```python
from build123d import *

# Parameters (mm, degrees)
F0_R     = 1.6002
F1_DEPTH = 6.35


with BuildPart() as f1:
    # F0 (on Right) → F1 (new body)
    with BuildSketch(Plane.YZ):
        Polygon((6.35, 0), (-6.35, 0), (-6.35, 6.604), (-21.59, 6.604), (-21.59, -19.304), (-6.35, -19.304), (-6.35, -12.7), (6.35, -12.7), (6.35, -19.304), (21.59, -19.304), (21.59, 6.604), (6.35, 6.604), align=None)
        with Locations((-6.35, -6.35)):
            Circle(F0_R, mode=Mode.SUBTRACT)
    extrude(amount=F1_DEPTH)


solid = f1.part
```
The model under review builds one solid part; all positions refer to its coordinate system, in mm. A direction names the side the tool comes from. Round coordinates to 2 decimals unless told otherwise and drop trailing zeros. Write each loop counter-clockwise with the first axis right and the second up, starting at its lowest first coordinate (ties: lowest second). Pieces come first, ordered by that corner, then holes. Notation, with made-up numbers: (30.5, 67.25) -> (57.5, 67.25) arc R10 cw to (57.5, 81.25) -> close; hole circle Ø1 at (68, -30). An arc over 180 degrees is marked (long way). Use CSV: the item, a comma, the result in double quotes.
Q1. Mouldability with a two-part tool opening along Y and no side actions: class faces 4 (the flat face through (3, 14, -19.304)), 5 (the flat face through (3, -6.35, 3)), 6 (the flat face through (3, 21.59, -7)) as released by +Y, released by -Y, zero draft, split by the parting line, or undercut.
Checks:
face 4,"zero draft"
face 5,"undercut"
face 6,"released by +Y"
Q2. Consider section C-C (y = 5). Give the boundary of the cut face in (x, z), then the cut area to 3 significant figures.
Checks:
outline,"(0, -12.7) -> (6.35, -12.7) -> (6.35, 0) -> (0, 0) -> close"
area,"80.6 mm²"
Q3. Consider section B-B (x = 5.75). Give the boundary of the cut face in (y, z).
Checks:
outline,"(-21.59, -19.3) -> (-6.35, -19.3) -> (-6.35, -12.7) -> (6.35, -12.7) -> (6.35, -19.3) -> (21.59, -19.3) -> (21.59, 6.6) -> (6.35, 6.6) -> (6.35, 0) -> (-6.35, 0) -> (-6.35, 6.6) -> (-21.59, 6.6) -> close; hole circle Ø3.2 at (-6.35, -6.35)"
Q4. Consider section A-A (z = 0.75). Give the boundary of the cut face in (x, y), then the cut area to 3 significant figures.
Checks:
outline,"(0, -21.59) -> (6.35, -21.59) -> (6.35, -6.35) -> (0, -6.35) -> close; (0, 6.35) -> (6.35, 6.35) -> (6.35, 21.59) -> (0, 21.59) -> close"
area,"194 mm²"
Q5. For pin 1 Ø3 at (x, y) = (4, 0.5) entering from +Z; pin 2 Ø1.9 at (x, y) = (2.5, 1.5) entering from -Z, all flat-tipped, find the tip position at first contact; note any pin that passes through.
Checks:
pin 1,"z = 0"
pin 2,"z = -12.7"
Q6. For faces 1 (the flat face through (3, -21.59, -6)), 2 (the flat face through (3, 0, 0)), 3 (the flat face through (3, -6.35, -16)), list the 3-axis set-ups (+Z, -Z, +X, -X, +Y, -Y) from which the entire face can be reached by the end or side of a thin tool; tool diameter is ignored.
Checks:
face 1,"+Z, -Z, +X, -X, -Y"
face 2,"+Z, +X, -X"
face 3,"-Z, +X, -X"
Q7. Consider section D-D (z = -6.35). Give the boundary of the cut face in (x, y), then the cut area to 3 significant figures.
Checks:
outline,"(0, -21.59) -> (6.35, -21.59) -> (6.35, -7.95) -> (0, -7.95) -> close; (0, -4.75) -> (6.35, -4.75) -> (6.35, 21.59) -> (0, 21.59) -> close"
area,"254 mm²"
Q8. To check wall thickness, follow probe 1 along Y at (x, z) = (3.5, 5.25); probe 2 along Y at (x, z) = (2.25, -7); probe 3 along Z at (x, y) = (1.5, -1). State the ranges of each line that lie inside material, in increasing order. Write a range as [from, to].
Checks:
probe 1,"[-21.59, -6.35], [6.35, 21.59]"
probe 2,"[-21.59, -7.81], [-4.89, 21.59]"
probe 3,"[-12.7, 0]"
